from build123d import *

# Parameters (mm, degrees)
F0_W     = 48
F0_H     = 24.2
F0_R     = 1.6
F1_DEPTH = 1
F2_R     = 1.05
F3_DEPTH = 2.5
F2_R_2   = 2.1
F2_R_3   = 0.75
F4_DEPTH = 1.001
F5_W     = 5.6
F5_H     = 10
F6_DEPTH = 2.85
F2_W     = 4.3
F2_H     = 2.9
F7_DEPTH = 3.5


with BuildPart() as f1:
    # F0 (on Front) → F1 (new body)
    with BuildSketch(Plane.XZ):
        Rectangle(F0_W, F0_H)
        with Locations((-4.1, -2.4)):
            Circle(F0_R, mode=Mode.SUBTRACT)
        with Locations((9.7, 8.1)):
            Circle(F0_R, mode=Mode.SUBTRACT)
    extrude(amount=-F1_DEPTH)

    # F2 (on face) → F3 (join)
    with BuildSketch(Plane(origin=(0, 1, 0), x_dir=(-1, 0, 0), z_dir=(0, 1, 0))):
        with Locations((-11.4, 5.1)):
            Circle(F2_R)
    extrude(amount=F3_DEPTH)

    # F2 (on face) → F4 (cut, through all)
    with BuildSketch(Plane(origin=(0, 1, 0), x_dir=(-1, 0, 0), z_dir=(0, 1, 0))):
        with Locations((-21, 6.1)):
            Circle(F2_R_2)
        with Locations((-21, -8.9)):
            Circle(F2_R_2)
        with Locations((21, 6.1)):
            Circle(F2_R_2)
        with Locations((21, -8.9)):
            Circle(F2_R_2)
        with Locations((-3.7, 10.1)):
            Circle(F2_R_3)
    extrude(amount=-F4_DEPTH, mode=Mode.SUBTRACT)

    # F5 (on face) → F6 (join)
    with BuildSketch(Plane(origin=(0, 1, 0), x_dir=(-1, 0, 0), z_dir=(0, 1, 0))):
        with Locations((9.5, 7.1)):
            Rectangle(F5_W, F5_H)
    extrude(amount=F6_DEPTH)

    # F2 (on face) → F7 (join)
    with BuildSketch(Plane(origin=(0, 1, 0), x_dir=(-1, 0, 0), z_dir=(0, 1, 0))):
        with Locations((-5.65, -8.05)):
            Rectangle(F2_W, F2_H)
    extrude(amount=F7_DEPTH)


solid = f1.part
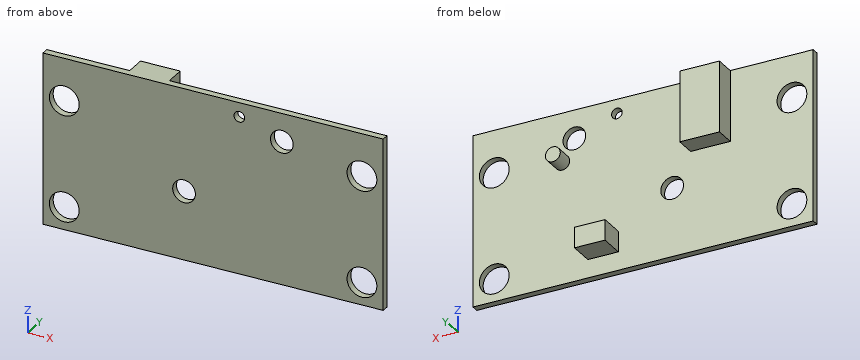
The listing builds one solid part. Answer for the finished solid, in the listing's coordinates (mm). Coordinates: 2 decimals unless noted, no trailing zeros. Write each loop counter-clockwise with the first axis right and the second up, starting at its lowest first coordinate (ties: lowest second). Pieces come first, ordered by that corner, then holes. Notation, with made-up numbers: M 74.5,35 L 79.5,35 A13 cw 79.5,43 Z; hole C 20.25,-25.75 d6. An arc over 180 degrees is marked long. Use one line per item in the form item = value.
Item 1: Find the intervals of material crossed by probe 1 along Z at (x, y) = (-21, 0.35); probe 2 along X at (y, z) = (0.85, -7.5); probe 3 along Z at (x, y) = (9.7, 0.4), in increasing order.
Model answer:
probe_1 = -12.1 to -11, -6.8 to 4, 8.2 to 12.1
probe_2 = -24 to -22.57, -19.43 to 19.43, 22.57 to 24
probe_3 = -12.1 to 6.5, 9.7 to 12.1
Item 2: Find section C-C, the plane x = 21. Give the vertices of the cut face in (y, z), plus the area to 3 significant figures.
Model answer:
outline = M 0,-12.1 L 1,-12.1 L 1,-11 L 0,-11 Z; M 0,-6.8 L 1,-6.8 L 1,4 L 0,4 Z; M 0,8.2 L 1,8.2 L 1,12.1 L 0,12.1 Z
area = 15.8 mm2
Item 3: Find section B-B, the plane y = 0.45. Give the vertices of the cut face in (x, z).
Model answer:
outline = M -24,-12.1 L 24,-12.1 L 24,12.1 L -24,12.1 Z; hole C -21,-8.9 d4.2; hole C -21,6.1 d4.2; hole C -4.1,-2.4 d3.2; hole C 3.7,10.1 d1.5; hole C 9.7,8.1 d3.2; hole C 21,-8.9 d4.2; hole C 21,6.1 d4.2
Item 4: Given P1, Ø2, axis at x = 7, y = 3, coming from the +Z side; P2, Ø3, axis at x = 17.5, z = 2, coming from the +Y side; P3, Ø3, axis at x = -10, z = 6, coming from the +Y side; P4, Ø1, axis at x = -18.5, z = -5, coming from the -Y side, each flat-ended and moving along its own axis, determine where each tip first touches the part or whether it passes through.
Model answer:
P1 = -6.6
P2 = 1
P3 = 3.85
P4 = 0
Item 5: Find section D-D, the plane z = 5.1. Give the vertices of the cut face in (x, y), plus the area to 3 significant figures.
Model answer:
outline = M -24,0 L -22.85,0 L -22.85,1 L -24,1 Z; M -19.15,0 L 19.15,0 L 19.15,1 L 12.45,1 L 12.45,3.5 L 10.35,3.5 L 10.35,1 L -6.7,1 L -6.7,3.85 L -12.3,3.85 L -12.3,1 L -19.15,1 Z; M 22.85,0 L 24,0 L 24,1 L 22.85,1 Z
area = 61.8 mm2
Item 6: Find section A-A, the plane x = -4.1. Give the vertices of the cut face in (y, z), plus the area to 3 significant figures.
Model answer:
outline = M 0,-12.1 L 1,-12.1 L 1,-4 L 0,-4 Z; M 0,-0.8 L 1,-0.8 L 1,12.1 L 0,12.1 Z
area = 21.0 mm2
